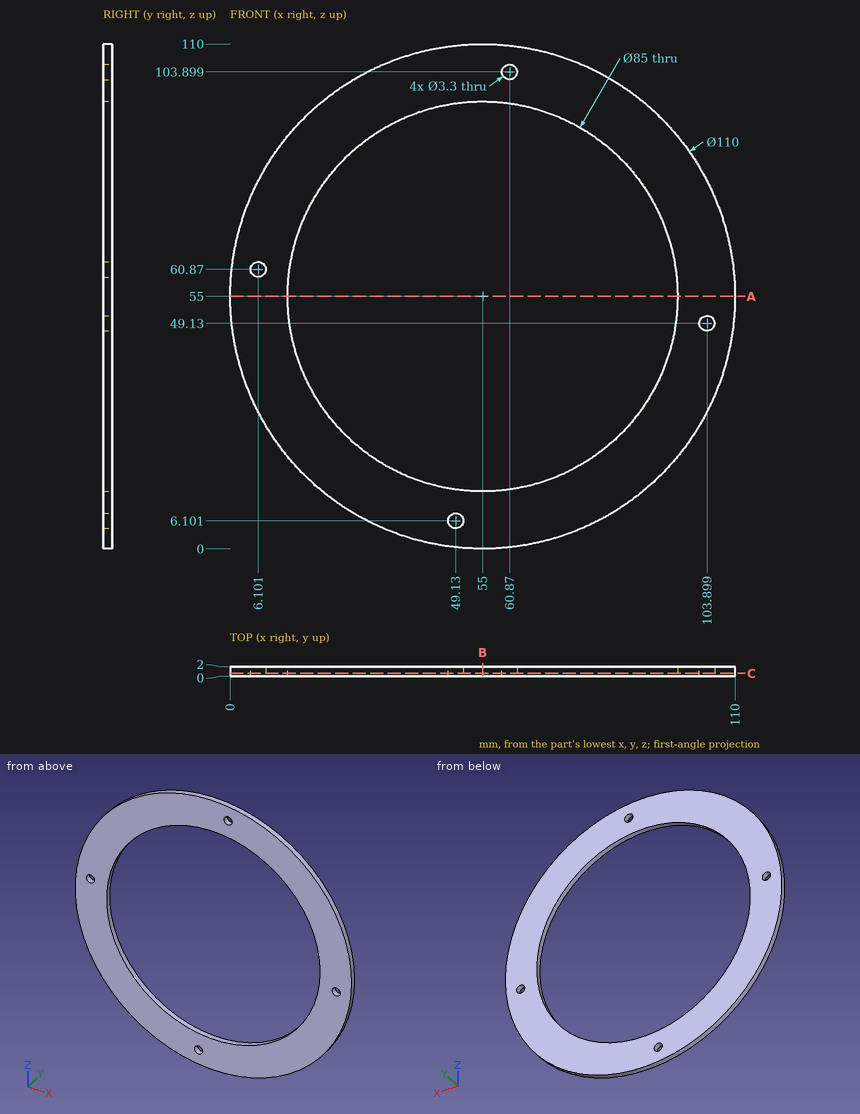
Can you work these out from the drawing? Everything is in mm from the part's minimum corner. Round coordinates to 2 decimals unless told otherwise and drop trailing zeros. Order: outer loops, then holes, each group sorted by start corner. A loop starts at its lowest first (then second) coordinate and runs counter-clockwise, first axis right, second up.
(1) If I drill on L1, parallel to Z at x = 61, y = 0.6 (1 decimal); L2, parallel to X at y = 1.15, z = 55, over which ranges is the centre line in solid material (lowest first)?
Results are:
L1: z = 0.3 to 12.9, 97.1 to 102.3, 105.5 to 109.7
L2: x = 0 to 12.5, 97.5 to 110
(2) If we section it at A-A (z = 55): Please give me the cut outline in (x, y).
Results are:
outline: (0, 0) - (12.5, 0) - (12.5, 2) - (0, 2) - close; (97.5, 0) - (110, 0) - (110, 2) - (97.5, 2) - close
(3) If we section it at C-C (y = 0.55): Please give me the cut outline in (x, z).
Results are:
outline: circle Ø110 at (55, 55); hole circle Ø3.3 at (6.1, 60.87); hole circle Ø85 at (55, 55); hole circle Ø3.3 at (49.13, 6.1); hole circle Ø3.3 at (60.87, 103.9); hole circle Ø3.3 at (103.9, 49.13)
(4) If we section it at B-B (x = 55): Please give me the cut outline in (y, z).
Results are:
outline: (0, 0) - (2, 0) - (2, 12.5) - (0, 12.5) - close; (0, 97.5) - (2, 97.5) - (2, 110) - (0, 110) - close
